Can you work these out from the model? Positions are in its coordinate system, mm. A direction names the side the tool comes from. Coordinates: 2 decimals unless noted, no trailing zeros. Loops run counter-clockwise (first coordinate to the right, second up) from the corner with the lowest first, then second, coordinate; pieces in that order, holes last. Notation, with made-up numbers: M 52,-24.75 L 105,-24.75 A12 ccw 105,-11.75 Z; hole C 47.25,-35 d7. An arc over 180 degrees is marked long. Answer as a JSON object with one key per item and string values. Group by question number.
Item 1: If I drill on line 1 (Z direction, x = 539.75, y = 4); line 2 (Z direction, x = 498.5, y = 1.5); line 3 (Z direction, x = 432.5, y = 4), over which ranges is the centre line in solid material (lowest first)?
Item 2: I'm going to push a flat-ended pin straight in: pin 1 Ø2.5 at (x, z) = (40.99, -196.85) entering from +Y. Where does the tip first touch, or does it pass through?
Item 3: Which directions (+Z, -Z, +X, -X, +Y, -Y) give clear straight access to the entire face, cutting with the end or side of a thin tool? Please do faces 4 (the flat face through (170, 3.81, -197)), 5 (the flat face through (394, 6.35, -166)).
Item 4: Suppose I cut it at A-A (x = 410). Write out the boundary of the cut face in (y, z).
Item 5: Suppose I cut it at B-B (y = 5). Count the separate pieces of the cut face and the enclosed holes in it, then the cut area to 3 significant figures.
Item 6: We'd pull the mould along X, two halves only. Please class faces 1 (the flat face through (399, 3.81, -197)), 2 (the flat face through (628, 3.81, -197)), 3 (the flat face through (394, 0, -212)): +X half, -X half, draft (parallel to the pull), parting line (faces both ways), or undercut.
```python
from build123d import *

# Parameters (mm, degrees)
SKETCH1_W               = 800.1
SKETCH1_H               = 419.1
BOSS_EXTRUDE1_DEPTH     = 6.35
SKETCH6_W               = 12.7
SKETCH6_H               = 419.1
BOSS_EXTRUDE2_DEPTH     = 6.35
CUT_EXTRUDE1_DEPTH      = 915.510236411
CUT_EXTRUDE1_DEPTH_BACK = 915.510236411
SKETCH4_R               = 1.1303
SKETCH5_R               = 1.1303
CUT_EXTRUDE2_DEPTH      = 915.510236411
SKETCH7_W               = 152.4
SKETCH7_H               = 50.8
CUT_EXTRUDE3_DEPTH      = 2.54
SKETCH8_R               = 0.889
CUT_EXTRUDE5_DEPTH      = 915.496126892
SKETCH9_R               = 0.889
CUT_EXTRUDE6_DEPTH      = 915.510236411
SKETCH10_R              = 0.889
CUT_EXTRUDE7_DEPTH      = 915.510236411


with BuildPart() as part:
    # Sketch1 → Boss-Extrude1 (new body)
    with BuildSketch(Plane(origin=(0, 0, 0), x_dir=(1, 0, 0), z_dir=(0, 1, 0))):
        with Locations((400.05, 209.55)):
            Rectangle(SKETCH1_W, SKETCH1_H)
    extrude(amount=BOSS_EXTRUDE1_DEPTH)

    # Sketch6 → Boss-Extrude2 (add)
    with BuildSketch(Plane(origin=(0, 6.35, 0), x_dir=(1, 0, 0), z_dir=(0, 1, 0))):
        with Locations((-6.35, 209.55)):
            Rectangle(SKETCH6_W, SKETCH6_H)
        with Locations((806.45, 209.55)):
            Rectangle(SKETCH6_W, SKETCH6_H)
    extrude(amount=-BOSS_EXTRUDE2_DEPTH)

    # Sketch4 → Cut-Extrude1 (cut, two sides: drawn at the far end of the back side and taken through both)
    with BuildSketch(Plane(origin=(0, 6.35, 0), x_dir=(1, 0, 0), z_dir=(0, 1, 0)).offset(-CUT_EXTRUDE1_DEPTH_BACK)):
        with Locations(Location((92.075, 390.525, 0), (0, 0, 270))):
            Circle(SKETCH4_R)
        with Locations(Location((250.825, 231.775, 0), (0, 0, 90))):
            Circle(SKETCH4_R)
        with Locations(Location((250.825, 390.525, 0), (0, 0, 270))):
            Circle(SKETCH4_R)
        with Locations(Location((92.075, 231.775, 0), (0, 0, 90))):
            Circle(SKETCH4_R)
        with Locations(Location((320.675, 390.525, 0), (0, 0, 270))):
            Circle(SKETCH4_R)
        with Locations(Location((320.675, 231.775, 0), (0, 0, 90))):
            Circle(SKETCH4_R)
        with Locations(Location((479.425, 231.775, 0), (0, 0, 90))):
            Circle(SKETCH4_R)
        with Locations(Location((479.425, 390.525, 0), (0, 0, 270))):
            Circle(SKETCH4_R)
        with Locations(Location((549.275, 390.525, 0), (0, 0, 270))):
            Circle(SKETCH4_R)
        with Locations(Location((549.275, 231.775, 0), (0, 0, 90))):
            Circle(SKETCH4_R)
        with Locations(Location((708.025, 231.775, 0), (0, 0, 90))):
            Circle(SKETCH4_R)
        with Locations(Location((708.025, 390.525, 0), (0, 0, 270))):
            Circle(SKETCH4_R)
        with Locations(Location((320.675, 161.925, 0), (0, 0, 270))):
            Circle(SKETCH4_R)
        with Locations(Location((320.675, 3.175, 0), (0, 0, 90))):
            Circle(SKETCH4_R)
        with Locations(Location((479.425, 3.175, 0), (0, 0, 90))):
            Circle(SKETCH4_R)
        with Locations(Location((479.425, 161.925, 0), (0, 0, 270))):
            Circle(SKETCH4_R)
        with Locations(Location((549.275, 161.925, 0), (0, 0, 270))):
            Circle(SKETCH4_R)
        with Locations(Location((549.275, 3.175, 0), (0, 0, 90))):
            Circle(SKETCH4_R)
        with Locations(Location((708.025, 3.175, 0), (0, 0, 90))):
            Circle(SKETCH4_R)
        with Locations(Location((708.025, 161.925, 0), (0, 0, 270))):
            Circle(SKETCH4_R)
        with Locations(Location((92.075, 161.925, 0), (0, 0, 270))):
            Circle(SKETCH4_R)
        with Locations(Location((92.075, 3.175, 0), (0, 0, 90))):
            Circle(SKETCH4_R)
        with Locations(Location((250.825, 3.175, 0), (0, 0, 90))):
            Circle(SKETCH4_R)
        with Locations(Location((250.825, 161.925, 0), (0, 0, 270))):
            Circle(SKETCH4_R)
    extrude(amount=CUT_EXTRUDE1_DEPTH + CUT_EXTRUDE1_DEPTH_BACK, mode=Mode.SUBTRACT)

    # Sketch5 → Cut-Extrude2 (cut, through all)
    with BuildSketch(Plane(origin=(0, 6.35, 0), x_dir=(1, 0, 0), z_dir=(0, 1, 0))):
        with Locations(Location((82.55, 95.25, 0), (0, 0, 270))):
            Circle(SKETCH5_R)
        with Locations(Location((31.75, 95.25, 0), (0, 0, 90))):
            Circle(SKETCH5_R)
        with Locations(Location((82.55, 298.45, 0), (0, 0, 90))):
            Circle(SKETCH5_R)
        with Locations(Location((31.75, 298.45, 0), (0, 0, 270))):
            Circle(SKETCH5_R)
        with Locations(Location((88.9, 196.85, 0), (0, 0, 270))):
            Circle(SKETCH5_R)
        with Locations(Location((25.4, 196.85, 0), (0, 0, 270))):
            Circle(SKETCH5_R)
        with Locations(Location((254, 196.85, 0), (0, 0, 270))):
            Circle(SKETCH5_R)
        with Locations(Location((317.5, 196.85, 0), (0, 0, 270))):
            Circle(SKETCH5_R)
        with Locations(Location((260.35, 95.25, 0), (0, 0, 90))):
            Circle(SKETCH5_R)
        with Locations(Location((311.15, 95.25, 0), (0, 0, 270))):
            Circle(SKETCH5_R)
        with Locations(Location((260.35, 298.45, 0), (0, 0, 270))):
            Circle(SKETCH5_R)
        with Locations(Location((311.15, 298.45, 0), (0, 0, 90))):
            Circle(SKETCH5_R)
        with Locations(Location((482.6, 196.85, 0), (0, 0, 270))):
            Circle(SKETCH5_R)
        with Locations(Location((546.1, 196.85, 0), (0, 0, 270))):
            Circle(SKETCH5_R)
        with Locations(Location((488.95, 95.25, 0), (0, 0, 90))):
            Circle(SKETCH5_R)
        with Locations(Location((539.75, 95.25, 0), (0, 0, 270))):
            Circle(SKETCH5_R)
        with Locations(Location((488.95, 298.45, 0), (0, 0, 270))):
            Circle(SKETCH5_R)
        with Locations(Location((539.75, 298.45, 0), (0, 0, 90))):
            Circle(SKETCH5_R)
        with Locations(Location((711.2, 196.85, 0), (0, 0, 270))):
            Circle(SKETCH5_R)
        with Locations(Location((774.7, 196.85, 0), (0, 0, 270))):
            Circle(SKETCH5_R)
        with Locations(Location((717.55, 95.25, 0), (0, 0, 90))):
            Circle(SKETCH5_R)
        with Locations(Location((768.35, 95.25, 0), (0, 0, 270))):
            Circle(SKETCH5_R)
        with Locations(Location((717.55, 298.45, 0), (0, 0, 270))):
            Circle(SKETCH5_R)
        with Locations(Location((768.35, 298.45, 0), (0, 0, 90))):
            Circle(SKETCH5_R)
    extrude(amount=-CUT_EXTRUDE2_DEPTH, mode=Mode.SUBTRACT)

    # Sketch7 → Cut-Extrude3 (cut)
    with BuildSketch(Plane(origin=(0, 6.35, 0), x_dir=(1, 0, 0), z_dir=(0, 1, 0))):
        with Locations((171.45, 196.85)):
            Rectangle(SKETCH7_W, SKETCH7_H)
        with Locations((400.05, 196.85)):
            Rectangle(SKETCH7_W, SKETCH7_H)
        with Locations((628.65, 196.85)):
            Rectangle(SKETCH7_W, SKETCH7_H)
    extrude(amount=-CUT_EXTRUDE3_DEPTH, mode=Mode.SUBTRACT)

    # Sketch8 → Cut-Extrude5 (cut, through all)
    with BuildSketch(Plane(origin=(0, 3.81, 0), x_dir=(1, 0, 0), z_dir=(0, 1, 0))):
        with Locations(Location((337.768946, 179.451, 0), (0, 0, 270))):
            Circle(SKETCH8_R)
        with Locations(Location((566.368946, 179.451, 0), (0, 0, 270))):
            Circle(SKETCH8_R)
        with Locations(Location((671.449, 196.469, 0), (0, 0, 270))):
            Circle(SKETCH8_R)
        with Locations(Location((214.249, 196.469, 0), (0, 0, 270))):
            Circle(SKETCH8_R)
        with Locations(Location((109.168946, 179.451, 0), (0, 0, 270))):
            Circle(SKETCH8_R)
        with Locations(Location((442.849, 196.469, 0), (0, 0, 270))):
            Circle(SKETCH8_R)
    extrude(amount=-CUT_EXTRUDE5_DEPTH, mode=Mode.SUBTRACT)

    # Sketch9 → Cut-Extrude6 (cut, through all)
    with BuildSketch(Plane(origin=(0, 6.35, 0), x_dir=(1, 0, 0), z_dir=(0, 1, 0))):
        with Locations(Location((40.985567, 196.85, 0), (0, 0, 270))):
            Circle(SKETCH9_R)
        with Locations(Location((57.15, 213.014433, 0), (0, 0, 270))):
            Circle(SKETCH9_R)
        with Locations(Location((73.314433, 196.85, 0), (0, 0, 270))):
            Circle(SKETCH9_R)
        with Locations(Location((57.15, 180.685567, 0), (0, 0, 270))):
            Circle(SKETCH9_R)
        with Locations(Location((269.585567, 196.85, 0), (0, 0, 270))):
            Circle(SKETCH9_R)
        with Locations(Location((285.75, 213.014433, 0), (0, 0, 270))):
            Circle(SKETCH9_R)
        with Locations(Location((301.914433, 196.85, 0), (0, 0, 270))):
            Circle(SKETCH9_R)
        with Locations(Location((285.75, 180.685567, 0), (0, 0, 270))):
            Circle(SKETCH9_R)
        with Locations(Location((498.185567, 196.85, 0), (0, 0, 270))):
            Circle(SKETCH9_R)
        with Locations(Location((514.35, 213.014433, 0), (0, 0, 270))):
            Circle(SKETCH9_R)
        with Locations(Location((530.514433, 196.85, 0), (0, 0, 270))):
            Circle(SKETCH9_R)
        with Locations(Location((514.35, 180.685567, 0), (0, 0, 270))):
            Circle(SKETCH9_R)
        with Locations(Location((726.785567, 196.85, 0), (0, 0, 270))):
            Circle(SKETCH9_R)
        with Locations(Location((742.95, 213.014433, 0), (0, 0, 270))):
            Circle(SKETCH9_R)
        with Locations(Location((759.114433, 196.85, 0), (0, 0, 270))):
            Circle(SKETCH9_R)
        with Locations(Location((742.95, 180.685567, 0), (0, 0, 270))):
            Circle(SKETCH9_R)
    extrude(amount=-CUT_EXTRUDE6_DEPTH, mode=Mode.SUBTRACT)

    # Sketch10 → Cut-Extrude7 (cut, through all)
    with BuildSketch(Plane(origin=(0, 6.35, 0), x_dir=(1, 0, 0), z_dir=(0, 1, 0))):
        with Locations(Location((45.296767183, 273.05, 0), (0, 0, 270))):
            Circle(SKETCH10_R)
        with Locations(Location((65.616767183, 273.05, 0), (0, 0, 90))):
            Circle(SKETCH10_R)
        with Locations(Location((65.616767183, 120.65, 0), (0, 0, 270))):
            Circle(SKETCH10_R)
        with Locations(Location((45.296767183, 120.65, 0), (0, 0, 90))):
            Circle(SKETCH10_R)
        with Locations(Location((273.896767183, 120.65, 0), (0, 0, 90))):
            Circle(SKETCH10_R)
        with Locations(Location((294.216767183, 120.65, 0), (0, 0, 270))):
            Circle(SKETCH10_R)
        with Locations(Location((273.896767183, 273.05, 0), (0, 0, 270))):
            Circle(SKETCH10_R)
        with Locations(Location((294.216767183, 273.05, 0), (0, 0, 90))):
            Circle(SKETCH10_R)
        with Locations(Location((502.496767183, 120.65, 0), (0, 0, 90))):
            Circle(SKETCH10_R)
        with Locations(Location((522.816767183, 120.65, 0), (0, 0, 270))):
            Circle(SKETCH10_R)
        with Locations(Location((502.496767183, 273.05, 0), (0, 0, 270))):
            Circle(SKETCH10_R)
        with Locations(Location((522.816767183, 273.05, 0), (0, 0, 90))):
            Circle(SKETCH10_R)
        with Locations(Location((731.096767183, 120.65, 0), (0, 0, 90))):
            Circle(SKETCH10_R)
        with Locations(Location((751.416767183, 120.65, 0), (0, 0, 270))):
            Circle(SKETCH10_R)
        with Locations(Location((731.096767183, 273.05, 0), (0, 0, 270))):
            Circle(SKETCH10_R)
        with Locations(Location((751.416767183, 273.05, 0), (0, 0, 90))):
            Circle(SKETCH10_R)
    extrude(amount=-CUT_EXTRUDE7_DEPTH, mode=Mode.SUBTRACT)


solid = part.part
```
From the geometry:
{
 "1": {"line 1": "-419.1 to -299.58, -297.32 to -96.38, -94.12 to 0", "line 2": "-419.1 to -197.68, -196.02 to 0", "line 3": "-419.1 to -222.25, -171.45 to 0"},
 "2": {"pin 1": "y = 6.35"},
 "3": {"face 4": "+Y", "face 5": "+Z, -Z, +X, -X, +Y"},
 "4": {"outline": "M 0,-419.1 L 6.35,-419.1 L 6.35,-222.25 L 3.81,-222.25 L 3.81,-171.45 L 6.35,-171.45 L 6.35,0 L 0,0 Z"},
 "5": {"separate pieces": "1", "enclosed holes": "83", "area": "322,000 mm2"},
 "6": {"face 1": "undercut", "face 2": "undercut", "face 3": "draft"}
}
